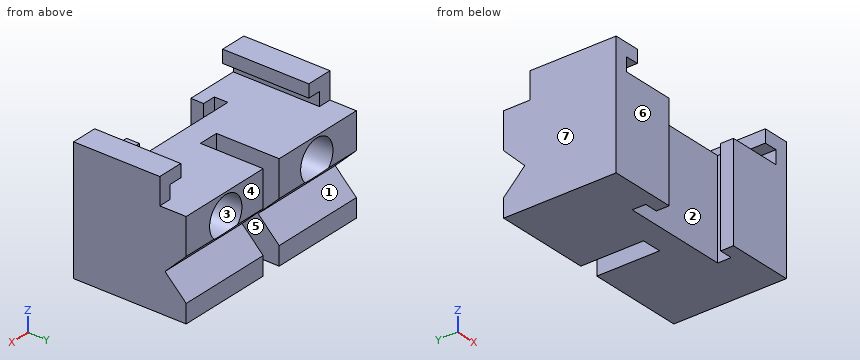
from build123d import *

# Parameters (mm, degrees)
CROQUIS1_W              = 50.8
CROQUIS1_H              = 27.051
SALIENTE_EXTRUIR1_DEPTH = 29.591
CORTAR_EXTRUIR1_DEPTH   = 42.295883595
CROQUIS8_W              = 4.7752
CROQUIS8_H              = 15.0876
CORTAR_EXTRUIR2_DEPTH   = 42.295883595
CORTAR_EXTRUIR3_DEPTH   = 48.472095113
CROQUIS12_R             = 4.826
CORTAR_EXTRUIR4_DEPTH   = 15.875
CROQUIS13_W             = 6.35
CROQUIS13_H             = 6.35
CORTAR_EXTRUIR5_DEPTH   = 61.330540106
CORTAR_EXTRUIR6_DEPTH   = 61.330540106


with BuildPart() as part:
    # Croquis1 → Saliente-Extruir1 (new body)
    with BuildSketch(Plane.XY):
        with Locations((-0.020777573, -0.020967748)):
            Rectangle(CROQUIS1_W, CROQUIS1_H)
    extrude(amount=SALIENTE_EXTRUIR1_DEPTH)

    # Croquis7 → Cortar-Extruir1 (cut, through all)
    with BuildSketch(Plane(origin=(0, 0, 0), x_dir=(-1, 0, 0), z_dir=(0, 0, -1))):
        Polygon((-12.7635, -7.196467748), (12.7635, -7.196467748), (12.7635, -10.447667748), (9.5885, -10.447667748), (9.5885, -13.546467748), (-9.5885, -13.546467748), (-9.5885, -10.447667748), (-12.7635, -10.447667748), align=None)
    extrude(amount=-CORTAR_EXTRUIR1_DEPTH, mode=Mode.SUBTRACT)

    # Croquis8 → Cortar-Extruir2 (cut, through all)
    with BuildSketch(Plane(origin=(0, 0, 0), x_dir=(-1, 0, 0), z_dir=(0, 0, -1))):
        with Locations((0, 5.960732252)):
            Rectangle(CROQUIS8_W, CROQUIS8_H)
    extrude(amount=-CORTAR_EXTRUIR2_DEPTH, mode=Mode.SUBTRACT)

    # Croquis9 → Cortar-Extruir3 (cut, through all)
    with BuildSketch(Plane(origin=(0, 13.504532252, 0), x_dir=(1, 0, 0), z_dir=(0, 1, 0))):
        Polygon((-19.1135, -29.591), (19.1135, -29.591), (19.1135, -26.4922), (22.2885, -26.4922), (22.2885, -23.241), (-22.2885, -23.241), (-22.2885, -26.4922), (-19.1135, -26.4922), align=None)
    extrude(amount=-CORTAR_EXTRUIR3_DEPTH, mode=Mode.SUBTRACT)

    # Croquis12 → Cortar-Extruir4 (cut)
    with BuildSketch(Plane(origin=(0, 13.504532252, 0), x_dir=(1, 0, 0), z_dir=(0, 1, 0))):
        with Locations(Location((-13.609777573, -17.8562, 0), (0, 0, 270))):
            Circle(CROQUIS12_R)
        with Locations(Location((13.568222427, -17.8562, 0), (0, 0, 270))):
            Circle(CROQUIS12_R)
    extrude(amount=-CORTAR_EXTRUIR4_DEPTH, mode=Mode.SUBTRACT)

    # Croquis13 → Cortar-Extruir5 (cut, through all)
    with BuildSketch(Plane(origin=(25.379222427, 0, 0), x_dir=(0, 0, -1), z_dir=(1, 0, 0))):
        with Locations((-26.416, 10.329532252)):
            Rectangle(CROQUIS13_W, CROQUIS13_H)
    extrude(amount=-CORTAR_EXTRUIR5_DEPTH, mode=Mode.SUBTRACT)

    # Croquis14 → Cortar-Extruir6 (cut, through all)
    with BuildSketch(Plane(origin=(25.379222427, 0, 0), x_dir=(0, 0, -1), z_dir=(1, 0, 0))):
        Polygon((-9.525, 8.424532252), (-4.445, 13.504532252), (-14.605, 13.504532252), align=None)
    extrude(amount=-CORTAR_EXTRUIR6_DEPTH, mode=Mode.SUBTRACT)


solid = part.part
Model file for the job. Use its own axes, mm. Face numbers are marked on the shaded views. A direction names the side the tool comes from. Round coordinates to 2 decimals unless told otherwise and drop trailing zeros. Loops run counter-clockwise (first coordinate to the right, second up) from the corner with the lowest first, then second, coordinate; pieces in that order, holes last. Notation, with made-up numbers: (13.25, 7.5) -> (71.25, 7.5) arc R30 ccw to (71.25, 41.5) -> close; hole circle Ø3 at (30.5, -24.5). An arc over 180 degrees is marked (long way). Answer as CSV lines item,"result". Start each with the question number.
1) Tool access for the marked faces 1, 2, 3 and 4: list every direction of +Z, -Z, +X, -X, +Y, -Y with a clear straight run to the whole face (end or side of a thin tool).
2) Pin check, flat tips, straight feed: P1, Ø8.5, axis at x = 13.57, z = 17.86, coming from the +Y side; P2, Ø3, axis at x = 0.5, z = 6.5, coming from the -Y side; P3, Ø2.5, axis at x = 0.5, z = 6.5, coming from the +Y side. Stop position of each tip, or through.
3) Mould opens along X. For the marked faces 5, 6 and 7 say: +X half, -X half, draft (parallel to the pull), parting line (faces both ways), or undercut.
4) Slice it at B-B (z = 25). List the corners of the cut face in (x, y).
5) Slice it at A-A (y = -9.5). List the corners of the cut face in (x, z), plus the area to 3 significant figures.
6) Probe line 1 along X through (y, z) = (8, 1.5); line 2 along X through (y, z) = (3.25, 15.25); line 3 along X through (y, z) = (0, 24.75). List the from-to ranges inside material, lowest first.
7) Slice it at D-D (y = 9.5). List the corners of the cut face in (x, z).
8) Slice it at C-C (x = -5). List the corners of the cut face in (y, z) (3 decimals), plus the area to 3 significant figures.
Filled in:
1,face 1,"+X, -X, +Y"
1,face 2,"+Z, -Z"
1,face 3,"+Y"
1,face 4,"+Z, -Z, +X, -X, +Y"
2,P1,"stops at y = -2.37"
2,P2,"stops at y = -7.2"
2,P3,"stops at y = -1.58"
3,face 5,"undercut"
3,face 6,"draft"
3,face 7,"-X half"
4,outline,"(-25.42, -13.55) -> (-22.29, -13.55) -> (-22.29, 7.15) -> (-25.42, 7.15) -> close; (22.29, -13.55) -> (25.38, -13.55) -> (25.38, 7.15) -> (22.29, 7.15) -> close"
5,outline,"(-25.42, 0) -> (-12.76, 0) -> (-12.76, 23.24) -> (-22.29, 23.24) -> (-22.29, 26.49) -> (-19.11, 26.49) -> (-19.11, 29.59) -> (-25.42, 29.59) -> close; (12.76, 0) -> (25.38, 0) -> (25.38, 29.59) -> (19.11, 29.59) -> (19.11, 26.49) -> (22.29, 26.49) -> (22.29, 23.24) -> (12.76, 23.24) -> close"
5,area,"647 mm2"
6,line 1,"x = -25.42 to -2.39, 2.39 to 25.38"
6,line 2,"x = -25.42 to -17.67, -9.55 to -2.39, 2.39 to 9.51, 17.63 to 25.38"
6,line 3,"x = -25.42 to -22.29, 22.29 to 25.38"
7,outline,"(-25.42, 0) -> (-2.39, 0) -> (-2.39, 8.45) -> (-25.42, 8.45) -> close; (-25.42, 10.6) -> (-2.39, 10.6) -> (-2.39, 23.24) -> (-25.42, 23.24) -> close; (2.39, 0) -> (25.38, 0) -> (25.38, 8.45) -> (2.39, 8.45) -> close; (2.39, 10.6) -> (25.38, 10.6) -> (25.38, 23.24) -> (2.39, 23.24) -> close; hole circle Ø9.65 at (-13.61, 17.86); hole circle Ø9.65 at (13.57, 17.86)"
8,outline,"(-7.196, 0) -> (13.505, 0) -> (13.505, 4.445) -> (8.425, 9.525) -> (13.505, 14.605) -> (13.505, 23.241) -> (-7.196, 23.241) -> close"
8,area,"455 mm2"
